from build123d import *

# Parameters (mm, degrees)
BODY_ANGLE                  = 180
HOLE_FOR_HANDLE_DEPTH       = 7.5
SKETCH6_R                   = 1.1303
F_5_40_SET_SCREW_HOLE_DEPTH = 7
SKETCH8_R                   = 0.75
HOLE_FOR_CABLE_DEPTH        = 7
SKETCH9_R                   = 6.5
SKETCH9_R_2                 = 0.75
BOSS_EXTRUDE1_DEPTH         = 2
SKETCH10_R                  = 0.8
F_2X0_4_SCREW_HOLE_DEPTH    = 14
SKETCH11_R                  = 1
CUT_EXTRUDE5_DEPTH          = 4
SKETCH12_R                  = 1.875
CUT_EXTRUDE6_DEPTH          = 1.5
REVOLVE4_ANGLE              = 180
SKETCH14_R                  = 0.75
CUT_EXTRUDE7_DEPTH          = 7.5
SKETCH15_W                  = 12.911147491
SKETCH15_H                  = 21.852119754
CUT_EXTRUDE9_DEPTH          = 14.0000001


with BuildPart() as part:
    # Sketch3 → body (revolve)
    with BuildSketch(Plane.XY):
        with BuildLine():
            Line((0, 6.5), (0, -6.5))
            ThreePointArc((0, -6.5), (6.5, 0), (0, 6.5))
        make_face()
    revolve(axis=Axis((0, 6.5, 0), (0, -1, 0)), revolution_arc=BODY_ANGLE)

    # Sketch5 → hole for handle (cut, through all)
    with BuildSketch(Plane(origin=(0, 0, 0), x_dir=(-1, 0, 0), z_dir=(0, 0, -1))):
        with BuildLine():
            Line((1.5, 3.688881761), (1.5, 2.702827207))
            Line((1.5, 2.702827207), (-1.5, 2.702827207))
            Line((-1.5, 2.702827207), (-1.5, 3.688881761))
            Line((-1.5, 3.688881761), (-1.5, 3.788881761))
            ThreePointArc((-1.5, 3.788881761), (0, -4.075), (1.5, 3.788881761))
            Line((1.5, 3.788881761), (1.5, 3.688881761))
        make_face()
    extrude(amount=-HOLE_FOR_HANDLE_DEPTH, mode=Mode.SUBTRACT)

    # Sketch6 → 5-40 set screw hole (cut)
    with BuildSketch(Plane(origin=(0, 6.5, 0), x_dir=(1, 0, 0), z_dir=(0, 1, 0))):
        with Locations((0, -1.564027547)):
            Circle(SKETCH6_R)
    extrude(amount=-F_5_40_SET_SCREW_HOLE_DEPTH, mode=Mode.SUBTRACT)

    # Sketch8 → hole for cable (cut)
    with BuildSketch(Plane(origin=(0, 0, 0), x_dir=(-1, 0, 0), z_dir=(0, 0, -1))):
        with Locations((0, 4.237225844)):
            Circle(SKETCH8_R)
    extrude(amount=-HOLE_FOR_CABLE_DEPTH, mode=Mode.SUBTRACT)

    # Sketch9 → Boss-Extrude1 (add)
    with BuildSketch(Plane(origin=(0, 0, 0), x_dir=(-1, 0, 0), z_dir=(0, 0, -1))):
        Circle(SKETCH9_R)
        with Locations((0, 4.237225844)):
            Circle(SKETCH9_R_2, mode=Mode.SUBTRACT)
        with BuildLine():
            Line((-1.5, 2.702827207), (-1.5, 3.788881761))
            ThreePointArc((-1.5, 3.788881761), (0, -4.075), (1.5, 3.788881761))
            Line((1.5, 3.788881761), (1.5, 2.702827207))
            Line((1.5, 2.702827207), (-1.5, 2.702827207))
        make_face(mode=Mode.SUBTRACT)
    extrude(amount=BOSS_EXTRUDE1_DEPTH)

    # Sketch10 → 2X0.4 screw hole (cut, through all)
    with BuildSketch(Plane(origin=(6.5, 0, 0), x_dir=(0, 0, -1), z_dir=(1, 0, 0))):
        with Locations((-1.067713855, 0)):
            Circle(SKETCH10_R)
    extrude(amount=-F_2X0_4_SCREW_HOLE_DEPTH, mode=Mode.SUBTRACT)

    # Sketch11 → Cut-Extrude5 (cut)
    with BuildSketch(Plane(origin=(6.5, 0, 0), x_dir=(0, 0, -1), z_dir=(1, 0, 0))):
        with Locations((-1.067713855, 0)):
            Circle(SKETCH11_R)
    extrude(amount=-CUT_EXTRUDE5_DEPTH, mode=Mode.SUBTRACT)

    # Sketch12 → Cut-Extrude6 (cut)
    with BuildSketch(Plane(origin=(6.5, 0, 0), x_dir=(0, 0, -1), z_dir=(1, 0, 0))):
        with Locations((-1.067713855, 0)):
            Circle(SKETCH12_R)
    extrude(amount=-CUT_EXTRUDE6_DEPTH, mode=Mode.SUBTRACT)

    # Sketch13 → Revolve4 (revolve)
    with BuildSketch(Plane(origin=(0, 0, -2), x_dir=(-1, 0, 0), z_dir=(0, 0, -1))):
        with BuildLine():
            Line((0, 6.5), (0, -6.5))
            ThreePointArc((0, -6.5), (6.5, 0), (0, 6.5))
        make_face()
    revolve(axis=Axis((0, 6.5, -2), (0, -1, 0)), revolution_arc=REVOLVE4_ANGLE)

    # Sketch14 → Cut-Extrude7 (cut, through all)
    with BuildSketch(Plane.XY.offset(-2)):
        with Locations((0, 4.237225844)):
            Circle(SKETCH14_R)
        with BuildLine():
            Line((1.5, 3.788881761), (1.5, 2.702827207))
            Line((1.5, 2.702827207), (-1.5, 2.702827207))
            Line((-1.5, 2.702827207), (-1.5, 3.788881761))
            ThreePointArc((-1.5, 3.788881761), (0, -4.075), (1.5, 3.788881761))
        make_face()
    extrude(amount=-CUT_EXTRUDE7_DEPTH, mode=Mode.SUBTRACT)

    # Sketch15 → Cut-Extrude9 (cut, through all)
    with BuildSketch(Plane(origin=(0, 6.5, 0), x_dir=(1, 0, 0), z_dir=(0, 1, 0))):
        with Locations((-3.623390746, 1.595465377)):
            Rectangle(SKETCH15_W, SKETCH15_H)
    extrude(amount=-CUT_EXTRUDE9_DEPTH, mode=Mode.SUBTRACT)


solid = part.part
Check sheet for the modelled part. Datum: model origin and axes. Units: mm. A direction names the side the tool comes from. Give positions to 0.01 mm unless a question says otherwise; leave off trailing zeros. Loops run counter-clockwise (first coordinate to the right, second up) from the corner with the lowest first, then second, coordinate; pieces in that order, holes last. Notation, with made-up numbers: M -16.5,3 L 17.5,3 A15 ccw 17.5,12 Z; hole C -16,58 d6. An arc over 180 degrees is marked long. Use a Markdown table: item, result. Add a question column.
Q1. Sectioned sample at B-B, the plane x = 5.6. Record the cut outline in (y, z) (3 decimals), then the cut area to 3 significant figures.
Q2. Tool access check on faces 1 (the cylindrical face through (6.5, 0.1, -1)), 2 (the flat face through (5, -1, 0)). Record the directions out of +Z, -Z, +X, -X, +Y, -Y that give a thin tool (end or side, any length) a straight path to the whole face; none if there is none.
Q3. Sectioned sample at A-A, the plane y = 0. Record the cut outline in (x, z) (3 decimals), then the cut area to 3 significant figures.
Q4. Mould release check, pull along Z, two halves, no side actions. Record for faces 3 (the cylindrical face through (4.483, -0.383, 0.144)), 4 (the flat face through (2.832, -4, -1)): pulls with the +Z half, pulls with the -Z half, needs draft (parallel to the pull), parting line crosses it, or undercut.
Q5. Scan lines: line 1 along Y through (x, z) = (5.5, 1); line 2 along Z through (x, y) = (4.35, 0); line 3 along Z through (x, y) = (5.3, 0). Record each from-to range of solid material in increasing order. Write a range as [from, to].
Q6. Go/stop test with flat-tipped pins: pin 1 (4 mm diameter, centred on y = -4, z = -5.5, fed in from +X); pin 2 (2 mm diameter, centred on x = 5.5, z = 0, fed in from +Y); pin 3 (1.9 mm diameter, centred on y = -0.5, z = 1.5, fed in from +X). Record where each tip stops, or that it passes through.
Q7. Sectioned sample at C-C, the plane z = -4.75. Record the cut outline in (x, y) (3 decimals), then the cut area to 3 significant figures.
Q8. Sectioned sample at D-D, the plane x = 4.7. Record the cut outline in (y, z), then the cut area to 3 significant figures.
Verdict:
| question | item | result |
|---|---|---|
| 1 | outline | M -3.3,-2 A3.3 ccw 3.3,-2 L 3.3,0 A3.3 ccw -3.3,0 Z; hole C 0,1.068 d3.75 |
| 1 | area | 36.4 mm^2 |
| 2 | face 1 | +Z, -Z, +X |
| 2 | face 2 | +X |
| 3 | outline | M 4.075,-7.064 A6.5 ccw 6.5,-2 L 6.5,-0.807 L 5,-0.807 L 5,0.068 L 4.075,0.068 Z; M 4.075,2.068 L 5,2.068 L 5,2.943 L 5.796,2.943 A6.5 ccw 4.075,5.064 Z |
| 3 | area | 15.2 mm^2 |
| 4 | face 3 | undercut |
| 4 | face 4 | needs draft |
| 5 | line 1 | [-3.32, -1.87], [1.87, 3.32] |
| 5 | line 2 | [-6.83, 0.07], [2.07, 4.83] |
| 5 | line 3 | [-5.76, -0.81], [2.94, 3.76] |
| 6 | pin 1 | x = 5.59 |
| 6 | pin 2 | y = 4.69 |
| 6 | pin 3 | x = 5 |
| 7 | outline | M 2.832,-5.164 A5.89 ccw 2.832,5.164 L 2.832,2.93 A4.075 cw 2.832,-2.93 Z |
| 7 | area | 17.4 mm^2 |
| 8 | outline | M -4.49,-2 A4.49 ccw 4.49,-2 L 4.49,0 A4.49 ccw -4.49,0 Z; hole C 0,1.07 d2 |
| 8 | area | 78.2 mm^2 |
